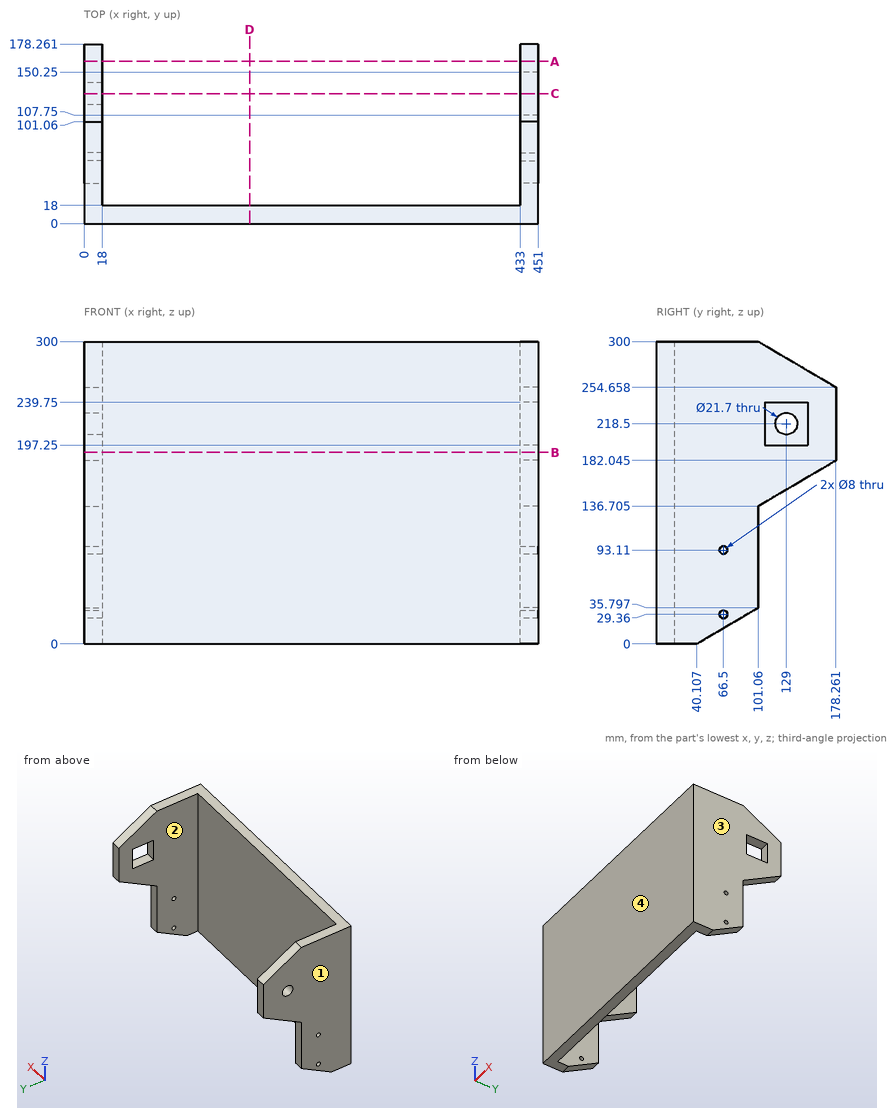
Can you work these out from the drawing? Everything is in mm from the part's minimum corner. Coordinates: 2 decimals unless noted, no trailing zeros. Loops run counter-clockwise (first coordinate to the right, second up) from the corner with the lowest first, then second, coordinate; pieces in that order, holes last. Notation, with made-up numbers: (15.25, 42.5) - (49.25, 42.5) arc R16 cw to (49.25, 60.5) - close; hole circle Ø6 at (-18.5, -34). An arc over 180 degrees is marked (long way). Put each result on its own line as item: value. Start each with the question number.
Item 1: Suppose I cut it at B-B (z = 190). Please give me the cut outline in (x, y).
Item 2: Suppose I cut it at A-A (y = 161). Please give me the cut outline in (x, z) (1 decimal).
Item 3: For pin 1 (5 mm diameter, centred on x = 387, z = 220, fed in from +Y); pin 2 (5.5 mm diameter, centred on x = 6, z = 94.5, fed in from +Y); pin 3 (20 mm diameter, centred on x = 438, y = 126, fed in from -Z), each with a flat end and sliding along its axis, tell me the tip position at first contact or that it passes through.
Item 4: Suppose I cut it at D-D (x = 164.5). Please give me the cut outline in (y, z), and give its area (3 significant figures).
Item 5: If I drill on line 1 along X through (y, z) = (35, 285.5); line 2 along Z through (x, y) = (8, 66) (1 decimal); line 3 along Y through (x, z) = (6, 93.11), over which ranges is the centre line in solid material (lowest first)?
Item 6: Suppose I cut it at C-C (y = 129). Please give me the cut outline in (x, z).
Item 7: If we mould it in two halves opening along X, with no side actions, what happens to the marked faces 1, 2, 3 and 4? For each: +X half, -X half, draft (parallel to the pull), parting line (faces both ways), or undercut.
Here are the results:
1. outline: (0, 0) - (451, 0) - (451, 178.26) - (433, 178.26) - (433, 18) - (18, 18) - (18, 178.26) - (0, 178.26) - close
2. outline: (0, 171.9) - (18, 171.9) - (18, 264.8) - (0, 264.8) - close; (433, 171.9) - (451, 171.9) - (451, 264.8) - (433, 264.8) - close
3. pin 1: y = 18
3. pin 2: y = 101.06
3. pin 3: z = 145.48
4. outline: (0, 0) - (18, 0) - (18, 300) - (0, 300) - close
4. area: 5,400 mm²
5. line 1: 0 to 18, 433 to 451
5. line 2: 15.2 to 25.4, 33.3 to 89.1, 97.1 to 300
5. line 3: 0 to 62.5, 70.5 to 101.06
6. outline: (0, 153.11) - (18, 153.11) - (18, 207.65) - (0, 207.65) - close; (0, 229.35) - (18, 229.35) - (18, 283.59) - (0, 283.59) - close; (433, 153.11) - (451, 153.11) - (451, 197.25) - (433, 197.25) - close; (433, 239.75) - (451, 239.75) - (451, 283.59) - (433, 283.59) - close
7. face 1: -X half
7. face 2: undercut
7. face 3: +X half
7. face 4: draft
